from build123d import *

# Parameters (mm, degrees)
SKETCH1_W                             = 120
SKETCH1_H                             = 100
BOTTOM_DEPTH                          = 3.5
SKETCH3_W                             = 120
SKETCH3_H                             = 100
WALL_DEPTH                            = 40
SKETCH4_R                             = 1.65
TOP_PLATE_SCREW_HOLES_DEPTH           = 30
TOP_PLATE_SCREW_HOLES_DRAFT           = -1
TOP_PLATE_SCREW_HOLES_PROFILE_2_DEPTH = 30
TOP_PLATE_SCREW_HOLES_PROFILE_2_DRAFT = -1
TOP_PLATE_SCREW_HOLES_PROFILE_3_DEPTH = 30
TOP_PLATE_SCREW_HOLES_PROFILE_3_DRAFT = -1
TOP_PLATE_SCREW_HOLES_PROFILE_4_DEPTH = 30
TOP_PLATE_SCREW_HOLES_PROFILE_4_DRAFT = -1
FILLET1_R                             = 2
FILLET2_R                             = 2
FILLET3_R                             = 2
FILLET4_R                             = 2
FILLET5_R                             = 2
FILLET6_R                             = 2
FILLET7_R                             = 2
FILLET8_R                             = 2
M4_MOUNT_R                            = 2.1
M4_MOUNT_CUT_DEPTH                    = 88.749643874
SKETCH7_R                             = 7.5
USB_CABEL_CUT_DEPTH                   = 90.399384785
FILLET9_R                             = 1
FILLET10_R                            = 1


with BuildPart() as part:
    # Sketch1 → Bottom (new body)
    with BuildSketch(Plane(origin=(0, 0, 0), x_dir=(1, 0, 0), z_dir=(0, 1, 0))):
        Rectangle(SKETCH1_W, SKETCH1_H)
    extrude(amount=BOTTOM_DEPTH)

    # Sketch3 → Wall (add)
    with BuildSketch(Plane(origin=(0, 3.5, 0), x_dir=(1, 0, 0), z_dir=(0, 1, 0))):
        Rectangle(SKETCH3_W, SKETCH3_H)
        Polygon((-51, 47), (51, 47), (51, 41), (57, 41), (57, -41), (51, -41), (51, -47), (-51, -47), (-51, -41), (-57, -41), (-57, 41), (-51, 41), align=None, mode=Mode.SUBTRACT)
    extrude(amount=WALL_DEPTH)


with BuildPart() as top_plate_screw_holes_tool:
    # Sketch4 → Top Plate Screw Holes (with draft: the straight prism first)
    with BuildSketch(Plane(origin=(0, 43.5, 0), x_dir=(1, 0, 0), z_dir=(0, 1, 0))):
        with Locations((-55, 45)):
            Circle(SKETCH4_R)
    extrude(amount=-TOP_PLATE_SCREW_HOLES_DEPTH)
    # Top Plate Screw Holes: the draft: its side faces are tilted about the plane it starts from
    top_plate_screw_holes_sides = [top_plate_screw_holes_tool.faces().sort_by_distance(p)[0] for p in [
        (-56.65, 28.5, -45),
    ]]
    draft(top_plate_screw_holes_sides, Plane(origin=(0, 43.5, 0), x_dir=(1, 0, 0), z_dir=(0, 1, 0)), TOP_PLATE_SCREW_HOLES_DRAFT)


with BuildPart() as part_1:
    add(part.part)

    # Top Plate Screw Holes: cut by top_plate_screw_holes_tool
    add(top_plate_screw_holes_tool.part, mode=Mode.SUBTRACT)


with BuildPart() as top_plate_screw_holes_profile_2_tool:
    # Sketch4 → Top Plate Screw Holes profile 2 (with draft: the straight prism first)
    with BuildSketch(Plane(origin=(0, 43.5, 0), x_dir=(1, 0, 0), z_dir=(0, 1, 0))):
        with Locations((55, 45)):
            Circle(SKETCH4_R)
    extrude(amount=-TOP_PLATE_SCREW_HOLES_PROFILE_2_DEPTH)
    # Top Plate Screw Holes profile 2: the draft: its side faces are tilted about the plane it starts from
    top_plate_screw_holes_profile_2_sides = [top_plate_screw_holes_profile_2_tool.faces().sort_by_distance(p)[0] for p in [
        (53.35, 28.5, -45),
    ]]
    draft(top_plate_screw_holes_profile_2_sides, Plane(origin=(0, 43.5, 0), x_dir=(1, 0, 0), z_dir=(0, 1, 0)), TOP_PLATE_SCREW_HOLES_PROFILE_2_DRAFT)


with BuildPart() as part_2:
    add(part_1.part)

    # Top Plate Screw Holes profile 2: cut by top_plate_screw_holes_profile_2_tool
    add(top_plate_screw_holes_profile_2_tool.part, mode=Mode.SUBTRACT)


with BuildPart() as top_plate_screw_holes_profile_3_tool:
    # Sketch4 → Top Plate Screw Holes profile 3 (with draft: the straight prism first)
    with BuildSketch(Plane(origin=(0, 43.5, 0), x_dir=(1, 0, 0), z_dir=(0, 1, 0))):
        with Locations((55, -45)):
            Circle(SKETCH4_R)
    extrude(amount=-TOP_PLATE_SCREW_HOLES_PROFILE_3_DEPTH)
    # Top Plate Screw Holes profile 3: the draft: its side faces are tilted about the plane it starts from
    top_plate_screw_holes_profile_3_sides = [top_plate_screw_holes_profile_3_tool.faces().sort_by_distance(p)[0] for p in [
        (53.35, 28.5, 45),
    ]]
    draft(top_plate_screw_holes_profile_3_sides, Plane(origin=(0, 43.5, 0), x_dir=(1, 0, 0), z_dir=(0, 1, 0)), TOP_PLATE_SCREW_HOLES_PROFILE_3_DRAFT)


with BuildPart() as part_3:
    add(part_2.part)

    # Top Plate Screw Holes profile 3: cut by top_plate_screw_holes_profile_3_tool
    add(top_plate_screw_holes_profile_3_tool.part, mode=Mode.SUBTRACT)


with BuildPart() as top_plate_screw_holes_profile_4_tool:
    # Sketch4 → Top Plate Screw Holes profile 4 (with draft: the straight prism first)
    with BuildSketch(Plane(origin=(0, 43.5, 0), x_dir=(1, 0, 0), z_dir=(0, 1, 0))):
        with Locations((-55, -45)):
            Circle(SKETCH4_R)
    extrude(amount=-TOP_PLATE_SCREW_HOLES_PROFILE_4_DEPTH)
    # Top Plate Screw Holes profile 4: the draft: its side faces are tilted about the plane it starts from
    top_plate_screw_holes_profile_4_sides = [top_plate_screw_holes_profile_4_tool.faces().sort_by_distance(p)[0] for p in [
        (-56.65, 28.5, 45),
    ]]
    draft(top_plate_screw_holes_profile_4_sides, Plane(origin=(0, 43.5, 0), x_dir=(1, 0, 0), z_dir=(0, 1, 0)), TOP_PLATE_SCREW_HOLES_PROFILE_4_DRAFT)


with BuildPart() as part_4:
    add(part_3.part)

    # Top Plate Screw Holes profile 4: cut by top_plate_screw_holes_profile_4_tool
    add(top_plate_screw_holes_profile_4_tool.part, mode=Mode.SUBTRACT)

    # Fillet1
    fillet1_edges = [part_4.edges().sort_by_distance(p)[0] for p in [
        (-51, 23.5, 41),
    ]]
    fillet(fillet1_edges, radius=FILLET1_R)

    # Fillet2
    fillet2_edges = [part_4.edges().sort_by_distance(p)[0] for p in [
        (51, 23.5, 41),
    ]]
    fillet(fillet2_edges, radius=FILLET2_R)

    # Fillet3
    fillet3_edges = [part_4.edges().sort_by_distance(p)[0] for p in [
        (51, 23.5, -41),
    ]]
    fillet(fillet3_edges, radius=FILLET3_R)

    # Fillet4
    fillet4_edges = [part_4.edges().sort_by_distance(p)[0] for p in [
        (-51, 23.5, -41),
    ]]
    fillet(fillet4_edges, radius=FILLET4_R)

    # Fillet5
    fillet5_edges = [part_4.edges().sort_by_distance(p)[0] for p in [
        (-60, 21.75, -50),
    ]]
    fillet(fillet5_edges, radius=FILLET5_R)

    # Fillet6
    fillet6_edges = [part_4.edges().sort_by_distance(p)[0] for p in [
        (60, 21.75, -50),
    ]]
    fillet(fillet6_edges, radius=FILLET6_R)

    # Fillet7
    fillet7_edges = [part_4.edges().sort_by_distance(p)[0] for p in [
        (60, 21.75, 50),
    ]]
    fillet(fillet7_edges, radius=FILLET7_R)

    # Fillet8
    fillet8_edges = [part_4.edges().sort_by_distance(p)[0] for p in [
        (-60, 21.75, 50),
    ]]
    fillet(fillet8_edges, radius=FILLET8_R)

    # M4 Mount → M4 Mount Cut (cut, through all)
    with BuildSketch(Plane.XZ.offset(-3.5)):
        with Locations(Location((30, -20, 0), (0, 0, 270))):
            Circle(M4_MOUNT_R)
        with Locations(Location((30, 20, 0), (0, 0, 270))):
            Circle(M4_MOUNT_R)
        with Locations(Location((-30, 20, 0), (0, 0, 90))):
            Circle(M4_MOUNT_R)
        with Locations(Location((-30, -20, 0), (0, 0, 90))):
            Circle(M4_MOUNT_R)
    extrude(amount=M4_MOUNT_CUT_DEPTH, mode=Mode.SUBTRACT)

    # Cut-Extrude3 cone 1 section (through the dimple's axis) → Cut-Extrude3 (revolve, cut)
    with BuildSketch(Plane(origin=(30, 3.5, 20), x_dir=(0, 0, 1), z_dir=(1, 0, 0))):
        Polygon((0, 0), (3.75, 0), (0, 3.75), align=None)
    revolve(axis=Axis((30, 3.5, 20), (0, -1, 0)), mode=Mode.SUBTRACT)

    # Cut-Extrude3 cone 2 section (through the dimple's axis) → Cut-Extrude3 cone 2 (revolve, cut)
    with BuildSketch(Plane(origin=(30, 3.5, -20), x_dir=(0, 0, 1), z_dir=(1, 0, 0))):
        Polygon((0, 0), (3.75, 0), (0, 3.75), align=None)
    revolve(axis=Axis((30, 3.5, -20), (0, -1, 0)), mode=Mode.SUBTRACT)

    # Cut-Extrude3 cone 3 section (through the dimple's axis) → Cut-Extrude3 cone 3 (revolve, cut)
    with BuildSketch(Plane(origin=(-30, 3.5, -20), x_dir=(0, 0, 1), z_dir=(1, 0, 0))):
        Polygon((0, 0), (3.75, 0), (0, 3.75), align=None)
    revolve(axis=Axis((-30, 3.5, -20), (0, -1, 0)), mode=Mode.SUBTRACT)

    # Cut-Extrude3 cone 4 section (through the dimple's axis) → Cut-Extrude3 cone 4 (revolve, cut)
    with BuildSketch(Plane(origin=(-30, 3.5, 20), x_dir=(0, 0, 1), z_dir=(1, 0, 0))):
        Polygon((0, 0), (3.75, 0), (0, 3.75), align=None)
    revolve(axis=Axis((-30, 3.5, 20), (0, -1, 0)), mode=Mode.SUBTRACT)

    # Sketch7 → USB Cabel Cut (cut, through all)
    with BuildSketch(Plane.XZ):
        with Locations(Location((0, -25, 0), (0, 0, 270))):
            Circle(SKETCH7_R)
    extrude(amount=-USB_CABEL_CUT_DEPTH, mode=Mode.SUBTRACT)

    # Fillet9
    fillet9_edges = [part_4.edges().sort_by_distance(p)[0] for p in [
        (0, 0, -17.5),
    ]]
    fillet(fillet9_edges, radius=FILLET9_R)

    # Fillet10
    fillet10_edges = [part_4.edges().sort_by_distance(p)[0] for p in [
        (0, 3.5, -17.5),
    ]]
    fillet(fillet10_edges, radius=FILLET10_R)


solid = part_4.part
For this review, take the finished solid that the model builds, in its own axes (mm). A direction names the side the tool comes from. Round coordinates to 2 decimals unless told otherwise and drop trailing zeros. Loops run counter-clockwise (first coordinate to the right, second up) from the corner with the lowest first, then second, coordinate; pieces in that order, holes last. Notation, with made-up numbers: (82.25, -19) - (141.25, -19) arc R13 cw to (141.25, -2) - close; hole circle Ø3 at (32, 42). An arc over 180 degrees is marked (long way). One line per question, with ' | ' between items.
Q1. The part is to be moulded in two halves that separate along Z. For faces 3 (the flat face through (-1, 21, 50)), 4 (the flat face through (-1, 21, -50)), 5 (the flat face through (57, 23, -1)), say which applies: released by +Z, released by -Z, zero draft, split by the parting line, or undercut.
Taken from the geometry:
face 3: released by +Z | face 4: released by -Z | face 5: undercut
Q2. Take a section at C-C (y = 36). Give the boundary of the cut face in (x, z), and give its area (3 significant figures).
Taken from the geometry:
outline: (-60, -48) arc R2 ccw to (-58, -50) - (58, -50) arc R2 ccw to (60, -48) - (60, 48) arc R2 ccw to (58, 50) - (-58, 50) arc R2 ccw to (-60, 48) - close; hole (-57, -41) - (-53, -41) arc R2 cw to (-51, -43) - (-51, -47) - (51, -47) - (51, -43) arc R2 cw to (53, -41) - (57, -41) - (57, 41) - (53, 41) arc R2 cw to (51, 43) - (51, 47) - (-51, 47) - (-51, 43) arc R2 cw to (-53, 41) - (-57, 41) - close; hole circle Ø3.04 at (-55, -45); hole circle Ø3.04 at (-55, 45); hole circle Ø3.04 at (55, -45); hole circle Ø3.04 at (55, 45) | area: 1,390 mm²
Q3. Take a section at A-A (z = 20). Give the boundary of the cut face in (x, y), and give its area (3 significant figures).
Taken from the geometry:
outline: (-60, 0) - (-32.1, 0) - (-32.1, 1.85) - (-33.75, 3.5) - (-57, 3.5) - (-57, 43.5) - (-60, 43.5) - close; (-27.9, 0) - (27.9, 0) - (27.9, 1.85) - (26.25, 3.5) - (-26.25, 3.5) - (-27.9, 1.85) - close; (32.1, 0) - (60, 0) - (60, 43.5) - (57, 43.5) - (57, 3.5) - (33.75, 3.5) - (32.1, 1.85) - close | area: 625 mm²
Q4. Take a section at D-D (x = -42.5). Give the boundary of the cut face in (y, z), and give its area (3 significant figures).
Taken from the geometry:
outline: (0, -50) - (43.5, -50) - (43.5, -47) - (3.5, -47) - (3.5, 47) - (43.5, 47) - (43.5, 50) - (0, 50) - close | area: 590 mm²
Q5. For pin 1 (1.1 mm diameter, centred on x = 55.5, z = -45, fed in from +Y); pin 2 (5 mm diameter, centred on x = -30, z = 20, fed in from +Y); pin 3 (24 mm diameter, centred on x = 0, z = -25, fed in from -Y); pin 4 (5.5 mm diameter, centred on x = 30, z = 20, fed in from +Y), all flat-tipped, find the tip position at first contact; note any pin that passes through.
Taken from the geometry:
pin 1: stops at y = 13.5 | pin 2: stops at y = 2.25 | pin 3: stops at y = 0 | pin 4: stops at y = 2.5
Q6. Take a section at B-B (x = 30). Give the boundary of the cut face in (y, z).
Taken from the geometry:
outline: (0, -50) - (43.5, -50) - (43.5, -47) - (3.5, -47) - (3.5, -23.75) - (1.85, -22.1) - (0, -22.1) - close; (0, -17.9) - (1.85, -17.9) - (3.5, -16.25) - (3.5, 16.25) - (1.85, 17.9) - (0, 17.9) - close; (0, 22.1) - (1.85, 22.1) - (3.5, 23.75) - (3.5, 47) - (43.5, 47) - (43.5, 50) - (0, 50) - close
Q7. Tool access review of faces 1 (the flat face through (-51, 23, 45)), 2 (the cylindrical face through (28.137, 0.938, 19.031)): name each direction out of +Z, -Z, +X, -X, +Y, -Y from which nothing blocks a thin tool from reaching the whole face with its end or side.
Taken from the geometry:
face 1: +Y | face 2: +Y, -Y
Q8. For line 1 along Z through (x, y) = (30, 1.2); line 2 along X through (y, z) = (1, 20); line 3 along X through (y, z) = (4.5, 26.5), list the stretches that pass through material, from the lowest coordinate up. Write a range as [from, to].
Taken from the geometry:
line 1: z = [-50, -22.1], [-17.9, 17.9], [22.1, 50] | line 2: x = [-60, -32.1], [-27.9, 27.9], [32.1, 60] | line 3: x = [-60, -57], [57, 60]
